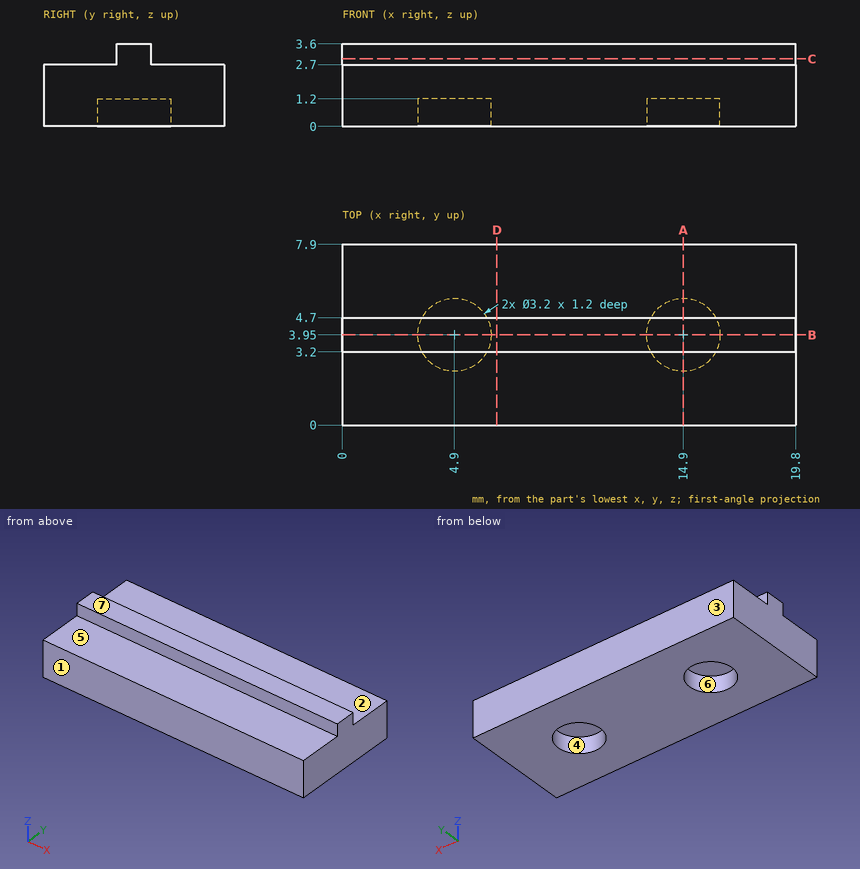
Input: dimensioned drawing with shaded views. Units: mm. Origin: part minimum x, y, z. A direction names the side the tool comes from. Coordinates: 2 decimals unless noted, no trailing zeros. Write each loop counter-clockwise with the first axis right and the second up, starting at its lowest first coordinate (ties: lowest second). Pieces come first, ordered by that corner, then holes. Notation, with made-up numbers: (74.5, -39.75) -> (105.5, -39.75) arc R22 cw to (105.5, -32.75) -> close; hole circle Ø5 at (4.5, -13). An arc over 180 degrees is marked (long way). Return JSON: item names as keys, results as strings. Group by question number.
1) Section query A-A, the plane x = 14.9. Return loops of the section in (y, z).
2) Ray query, line 1 along X through (y, z) = (3.95, 0.75); line 2 along X through (y, z) = (2.5, 0.4); line 3 along Z through (x, y) = (1.5, 2.5). Return the intervals inside material, ascending.
3) Section query B-B, the plane y = 3.95. Return loops of the section in (x, z), plus the area to 3 significant figures.
4) Section query D-D, the plane x = 6.75. Return loops of the section in (y, z).
5) Mould query, pull axis Y, two halves, no side actions, for the marked faces 1, 2, 3 and 4. Classes: +Y half, -Y half, draft (parallel to the pull), parting line (faces both ways), or undercut.
6) Section query C-C, the plane z = 2.95. Return loops of the section in (x, y).
7) Contact query for flat-ended pins moving along their axis: P1, Ø2.5, axis at x = 11, y = 7, coming from the +Z side; P2, Ø2, axis at y = 5.5, z = 3, coming from the +X side; P3, Ø1, axis at x = 5, y = 3.5, coming from the -Z side. Output: stop coordinate, or through.
8) Set-up query: the marked faces 5, 6 and 7. Return all of +Z, -Z, +X, -X, +Y, -Y with unobstructed straight access to the full face (end or side cutting, diameter ignored); none if empty.
From the geometry:
{
 "1": {"outline": "(0, 0) -> (2.35, 0) -> (2.35, 1.2) -> (5.55, 1.2) -> (5.55, 0) -> (7.9, 0) -> (7.9, 2.7) -> (4.7, 2.7) -> (4.7, 3.6) -> (3.2, 3.6) -> (3.2, 2.7) -> (0, 2.7) -> close"},
 "2": {"line 1": "0 to 3.3, 6.5 to 13.3, 16.5 to 19.8", "line 2": "0 to 4.22, 5.58 to 14.22, 15.58 to 19.8", "line 3": "0 to 2.7"},
 "3": {"outline": "(0, 0) -> (3.3, 0) -> (3.3, 1.2) -> (6.5, 1.2) -> (6.5, 0) -> (13.3, 0) -> (13.3, 1.2) -> (16.5, 1.2) -> (16.5, 0) -> (19.8, 0) -> (19.8, 3.6) -> (0, 3.6) -> close", "area": "63.6 mm²"},
 "4": {"outline": "(0, 0) -> (7.9, 0) -> (7.9, 2.7) -> (4.7, 2.7) -> (4.7, 3.6) -> (3.2, 3.6) -> (3.2, 2.7) -> (0, 2.7) -> close"},
 "5": {"face 1": "-Y half", "face 2": "draft", "face 3": "+Y half", "face 4": "undercut"},
 "6": {"outline": "(0, 3.2) -> (19.8, 3.2) -> (19.8, 4.7) -> (0, 4.7) -> close"},
 "7": {"P1": "z = 2.7", "P2": "x = 19.8", "P3": "z = 1.2"},
 "8": {"face 5": "+Z, +X, -X, -Y", "face 6": "-Z", "face 7": "+Z, +X, -X, +Y, -Y"}
}
